```python
from build123d import *

# Parameters (mm, degrees)
SKETCH1_W           = 64
SKETCH1_H           = 20
BOSS_EXTRUDE1_DEPTH = 48
BOSS_EXTRUDE2_DEPTH = 32
FILLET2_R           = 32
FILLET3_R           = 15


with BuildPart() as part:
    # Sketch1 → Boss-Extrude1 (new, symmetric)
    with BuildSketch(Plane.XY):
        Rectangle(SKETCH1_W, SKETCH1_H)
    extrude(amount=BOSS_EXTRUDE1_DEPTH, both=True)

    # Sketch1<3> → Boss-Extrude2 (add, symmetric)
    with BuildSketch(Plane.XY):
        Polygon((20, 10), (32, 10), (32, 73), (86.127416998, 127.127416998), (77.642135624, 135.612698372), (73.399494937, 131.370057685), (66.328427125, 124.298989873), (55.014718626, 112.985281374), (20, 77.970562748), align=None)
    extrude(amount=BOSS_EXTRUDE2_DEPTH, both=True)

    # Fillet2
    fillet2_edges = [part.edges().sort_by_distance(p)[0] for p in [
        (81.884776311, 131.370057685, -32),
        (81.884776311, 131.370057685, 32),
    ]]
    fillet(fillet2_edges, radius=FILLET2_R - 0.0001)  # a hair under: the kernel refuses the full size

    # Fillet3
    fillet3_edges = [part.edges().sort_by_distance(p)[0] for p in [
        (32, 73, 0),
        (20, 77.970562748, 0),
    ]]
    fillet(fillet3_edges, radius=FILLET3_R)

    # Sketch1<5> one side → Revolve3 (revolve)
    with BuildSketch(Plane.XY, mode=Mode.PRIVATE) as revolve3_sk:
        Polygon((66.328427125, 124.298989873), (55.014718626, 112.985281374), (63.5, 104.5), (86.127416998, 127.127416998), (77.642135624, 135.612698372), (73.399494937, 131.370057685), align=None)
        Polygon((66.328427125, 124.298989873), (73.399494937, 131.370057685), (50.384776311, 154.384776311), (43.313708499, 147.313708499), align=None)
    revolve(revolve3_sk.sketch.rotate(Axis((32, 136, 0), (0.7071067811865483, -0.7071067811865467, 0)), 180), axis=Axis((32, 136, 0), (0.7071067811865483, -0.7071067811865467, 0)))


solid = part.part
```
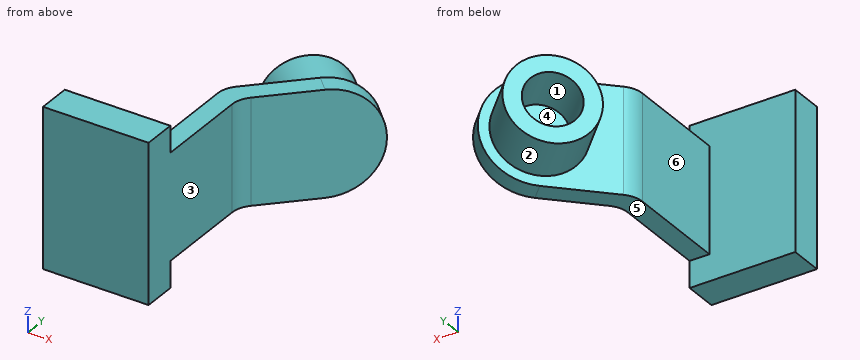
Geometry check sheet. Reference: the model listing, model coordinates, mm. Face numbers are marked on the shaded views. A direction names the side the tool comes from. Round coordinates to 2 decimals unless told otherwise and drop trailing zeros. Write each loop counter-clockwise with the first axis right and the second up, starting at its lowest first coordinate (ties: lowest second). Pieces come first, ordered by that corner, then holes. Notation, with made-up numbers: (81, 49.25) - (87, 49.25) arc R27 ccw to (87, 76.25) - close; hole circle Ø6 at (38.5, 46). An arc over 180 degrees is marked (long way). Write each question's results on one line, items separated by ' | '.
(1) Depth check by flat-ended pin: pin 1 Ø10 at (x, z) = (63.5, -17.5) entering from +Y; pin 2 Ø3 at (x, z) = (69, -11) entering from +Y; pin 3 Ø4 at (y, z) = (92.5, -23) entering from -X. Enter the tip coordinate at first touch or a pass-through.
Computed:
pin 1: stops at y = 139.06 | pin 2: stops at y = 134.09 | pin 3: stops at x = 32.53
(2) Set-up check for the marked faces 4, 5 and 6: record each of +Z, -Z, +X, -X, +Y, -Y from which the full face is reachable in a straight line by a thin tool's end or side.
Computed:
face 4: none | face 5: -Z, +X, -X, +Y | face 6: +Z, -Z, -X
(3) Thickness scan on probe 1 along X at (y, z) = (13, -31); probe 2 along Z at (x, y) = (39.5, 81.5); probe 3 along Y at (x, z) = (13, 23). Record the ranges inside material, lowest first. Write a range as from..to.
Computed:
probe 1: x = 20..32 | probe 2: z = -32..32 | probe 3: y = -10..10
(4) Sectioned sample at C-C, the plane z = 13. Enter the section's corners in (x, y), plus the area to 3 significant figures.
Computed:
outline: (-32, -10) - (32, -10) - (32, 66.79) arc R15 cw to (36.39, 77.39) - (84.18, 125.18) - (75.69, 133.66) - (70.94, 128.91) - (47.92, 151.92) - (38.6, 142.6) - (61.61, 119.58) - (48.42, 106.39) - (25.4, 129.4) - (16.08, 120.08) - (39.09, 97.06) - (24.39, 82.36) arc R15 ccw to (20, 71.76) - (20, 10) - (-32, 10) - close | area: 3,840 mm^2
(5) Sectioned sample at A-A, the plane z = -2.5. Enter the section's corners in (x, y).
Computed:
outline: (-32, -10) - (32, -10) - (32, 66.79) arc R15 cw to (36.39, 77.39) - (86.06, 127.06) - (77.57, 135.54) - (73.31, 131.28) - (50.3, 154.3) - (43.17, 147.17) - (66.19, 124.16) - (43.84, 101.81) - (20.83, 124.83) - (13.7, 117.7) - (36.72, 94.69) - (24.39, 82.36) arc R15 ccw to (20, 71.76) - (20, 10) - (-32, 10) - close
(6) Draft check along Z on the marked faces 1, 2 and 3. Enter one of: pulls with the +Z half, pulls with the -Z half, needs draft (parallel to the pull), parting line crosses it, or undercut.
Computed:
face 1: undercut | face 2: parting line crosses it | face 3: needs draft
(7) Sectioned sample at B-B, the plane y = 34.5. Enter the section's corners in (x, z), plus the area to 3 significant figures.
Computed:
outline: (20, -32) - (32, -32) - (32, 32) - (20, 32) - close | area: 768 mm^2
(8) Sectioned sample at D-D, the plane y = 6. Enter the section's corners in (x, z), plus the area to 3 significant figures.
Computed:
outline: (-32, -48) - (32, -48) - (32, 48) - (-32, 48) - close | area: 6,140 mm^2
